The listing builds one solid part. Answer for the finished solid, in the listing's coordinates (mm). Face numbers are marked on the shaded views. Round coordinates to 2 decimals unless told otherwise and drop trailing zeros. Loops run counter-clockwise (first coordinate to the right, second up) from the corner with the lowest first, then second, coordinate; pieces in that order, holes last. Notation, with made-up numbers: (27.5, -30) -> (37.5, -30) arc R17 ccw to (37.5, -7) -> close; hole circle Ø7 at (34, 66). An arc over 180 degrees is marked (long way). One line per question, with ' | ' between items.
from build123d import *

# Parameters (mm, degrees)
F0_R     = 22.75
F0_R_2   = 20.5
F1_DEPTH = 27.5
F2_R     = 2.8
F3_DEPTH = 25
F4_COUNT = 4
F4_ANGLE = 90


with BuildPart() as f1:
    # F0 (on Top) → F1 (new body)
    with BuildSketch(Plane.XY):
        Circle(F0_R)
        Circle(F0_R_2, mode=Mode.SUBTRACT)
    extrude(amount=F1_DEPTH)


with BuildPart() as f3:
    # F2 (on Right) → F3 (new body, symmetric)
    with BuildSketch(Plane.YZ):
        with Locations((0, 22.5)):
            Circle(F2_R)
    extrude(amount=F3_DEPTH, both=True)


with BuildPart() as f4_1:
    # F4: instance of F3
    add(f3.part.rotate(Axis((0, 0, 0), (0, 0, 1)), 1 * F4_ANGLE / (F4_COUNT - 1)))


with BuildPart() as f4_2:
    # F4: instance of F3
    add(f3.part.rotate(Axis((0, 0, 0), (0, 0, 1)), 2 * F4_ANGLE / (F4_COUNT - 1)))


with BuildPart() as f4_3:
    # F4: instance of F3
    add(f3.part.rotate(Axis((0, 0, 0), (0, 0, 1)), 3 * F4_ANGLE / (F4_COUNT - 1)))


with BuildPart() as f1_1:
    add(f1.part)

    # F5: cut F4_3, F4_2, F4_1, F3
    add(f4_3.part, mode=Mode.SUBTRACT)
    add(f4_2.part, mode=Mode.SUBTRACT)
    add(f4_1.part, mode=Mode.SUBTRACT)
    add(f3.part, mode=Mode.SUBTRACT)


solid = f1_1.part
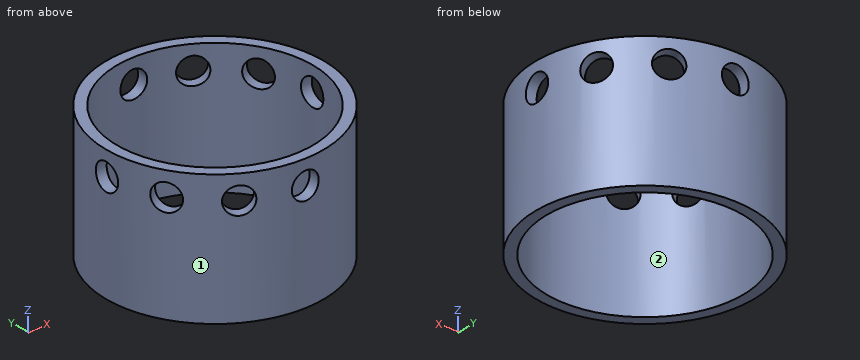
Q1. A cutting plane is placed at D-D on z = 22.5. Give the number of separate pieces and of enclosed holes in the cut face, plus the area to 3 significant figures.
Numbers:
separate pieces: 8 | enclosed holes: 0 | area: 205 mm^2
Q2. Given pin 1 Ø12 at (x, z) = (5.5, 22.5) entering from -Y; pin 2 Ø3 at (y, z) = (-9.5, 11.5) entering from -X; pin 3 Ø12 at (x, z) = (16.5, 23.5) entering from -Y; pin 4 Ø10 at (x, z) = (12, 9) entering from +Y, each flat-ended and moving along its own axis, determine where each tip first touches the part or whether it passes through.
Numbers:
pin 1: y = -22.75 | pin 2: x = -21.3 | pin 3: y = -20.18 | pin 4: y = 21.65
Q3. For a pull along X with two mould halves and no side action, classify the marked faces 1 and 2 as pulls with the +X half, pulls with the -X half, needs draft (parallel to the pull), parting line crosses it, or undercut.
Numbers:
face 1: parting line crosses it | face 2: undercut
Q4. A cutting plane is placed at A-A on y = 0. Give the vertices of the cut face in (x, z).
Numbers:
outline: (-22.75, 0) -> (-20.5, 0) -> (-20.5, 19.7) -> (-22.75, 19.7) -> close; (-22.75, 25.3) -> (-20.5, 25.3) -> (-20.5, 27.5) -> (-22.75, 27.5) -> close; (20.5, 0) -> (22.75, 0) -> (22.75, 19.7) -> (20.5, 19.7) -> close; (20.5, 25.3) -> (22.75, 25.3) -> (22.75, 27.5) -> (20.5, 27.5) -> close
Q5. A cutting plane is placed at C-C on y = 6.5. Give the vertices of the cut face in (x, z).
Numbers:
outline: (-21.8, 0) -> (-19.44, 0) -> (-19.44, 27.5) -> (-21.8, 27.5) -> close; (19.44, 0) -> (21.8, 0) -> (21.8, 27.5) -> (19.44, 27.5) -> close
Q6. Find the intervals of material crossed by line 1 (Z direction, x = 0, y = 22); line 2 (X direction, y = 0, z = 11), in increasing order. Write a range as from..to.
Numbers:
line 1: 0..19.7, 25.3..27.5 | line 2: -22.75..-20.5, 20.5..22.75
